The listing builds one solid part. Answer for the finished solid, in the listing's coordinates (mm). Coordinates: 2 decimals unless noted, no trailing zeros. Write each loop counter-clockwise with the first axis right and the second up, starting at its lowest first coordinate (ties: lowest second). Pieces come first, ordered by that corner, then holes.
(1) The part is cut by section A-A on z = 98. Give the number of separate pieces and of enclosed holes in the cut face, plus the area to 3 significant figures.
(2) The part is cut by section C-C on y = 48. Determine the outline of the cut face in (x, z).
(3) Straight lines are drawn through the part: line 1 (Y direction, x = 34.5, z = 41); line 2 (Z direction, x = 24, y = 36.5); line 3 (Y direction, x = -33, z = 49). For each, find the intervals that lie inside material, in ascending order.
(4) Given P1, Ø1.9, axis at x = 34, z = 52, coming from the -Y side; P2, Ø5, axis at x = 4, y = -36.5, coming from the -Z side; P3, Ø1.9, axis at x = 1, z = 97.5, coming from the +Y side, each flat-ended and moving along its own axis, determine where each tip first touches the part or whether it passes through.
(5) The part is cut by section B-B on x = 0. Determine the outline of the cut face in (y, z), plus the area to 3 significant figures.
Autodesk Fusion 360 part; units mm, degrees
sketch "Sketch1" plane through (0, 0, 0) normal (0, 0, 1) x (1, 0, 0)
  line L0 (63.5, 63.5) -> (-63.5, 63.5)
  line L1 (-63.5, 63.5) -> (-63.5, -63.5)
  line L2 (-63.5, -63.5) -> (63.5, -63.5)
  line L3 (63.5, -63.5) -> (63.5, 63.5)
  line L4 (63.5, 63.5) -> (-63.5, -63.5) construction
  line L5 (-63.5, 63.5) -> (63.5, -63.5) construction
extrude "Extrude1" add sketch "Sketch1" along normal blind 127
sketch "Sketch2" plane through (0, 0, 127) normal (0, 0, 1) x (-1, 0, 0)
  line L0 (-63.5, 63.5) -> (-63.5, -63.5)
  line L1 (-63.5, -63.5) -> (63.5, -63.5)
  line L2 (63.5, -63.5) -> (63.5, 63.5)
  line L3 (63.5, 63.5) -> (-63.5, 63.5)
  line L4 (31.75, 31.75) -> (-31.75, 31.75)
  line L5 (-31.75, 31.75) -> (-31.75, -31.75)
  line L6 (-31.75, -31.75) -> (31.75, -31.75)
  line L7 (31.75, -31.75) -> (31.75, 31.75)
  dimension "d3" = -31.75
sketch "Sketch3" plane through (0, -63.5, 0) normal (0, -1, 0) x (1, 0, 0)
  line L0 (-63.5, 0) -> (63.5, 0)
  line L1 (63.5, 0) -> (63.5, 127)
  line L2 (63.5, 127) -> (-63.5, 127)
  line L3 (-63.5, 127) -> (-63.5, 0)
  line L4 (-31.75, 31.75) -> (31.75, 31.75)
  line L5 (31.75, 31.75) -> (31.75, 95.25)
  line L6 (31.75, 95.25) -> (-31.75, 95.25)
  line L7 (-31.75, 95.25) -> (-31.75, 31.75)
  dimension "d4" = -31.75
sketch "Sketch4" plane through (0, 0, 0) normal (0, 0, -1) x (1, 0, 0)
  line L0 (63.5, -63.5) -> (63.5, 63.5)
  line L1 (63.5, 63.5) -> (-63.5, 63.5)
  line L2 (-63.5, 63.5) -> (-63.5, -63.5)
  line L3 (-63.5, -63.5) -> (63.5, -63.5)
sketch "Sketch5" plane through (-63.5, 0, 0) normal (-1, 0, 0) x (0, -1, 0)
  line L0 (-63.5, 0) -> (63.5, 0)
  line L1 (63.5, 0) -> (63.5, 127)
  line L2 (63.5, 127) -> (-63.5, 127)
  line L3 (-63.5, 127) -> (-63.5, 0)
  line L4 (-31.75, 31.75) -> (31.75, 31.75)
  line L5 (31.75, 31.75) -> (31.75, 95.25)
  line L6 (31.75, 95.25) -> (-31.75, 95.25)
  line L7 (-31.75, 95.25) -> (-31.75, 31.75)
  dimension "d5" = -31.75
extrude "Extrude2" cut sketch "Sketch2" against normal blind 127 contours L4 L5 L6 L7
extrude "Extrude3" cut sketch "Sketch5" against normal blind 127 contours L4 L5 L6 L7
extrude "Extrude4" cut sketch "Sketch3" against normal blind 127 contours L4 L5 L6 L7
chamfer "Chamfer1" distance 25.4 angle 45 4 edges at (0, -63.5, 95.25) (31.75, -63.5, 63.5) (0, -63.5, 31.75) (-31.75, -63.5, 63.5)
chamfer "Chamfer2" distance 25.4 angle 45 4 edges at (-63.5, 31.75, 63.5) (-63.5, 0, 95.25) (-63.5, -31.75, 63.5) (-63.5, 0, 31.75)
chamfer "Chamfer3" distance 25.4 angle 45 4 edges at (31.75, 63.5, 63.5) (0, 63.5, 95.25) (-31.75, 63.5, 63.5) (0, 63.5, 31.75)
chamfer "Chamfer4" distance 25.4 angle 45 4 edges at (63.5, 0, 95.25) (63.5, 31.75, 63.5) (63.5, 0, 31.75) (63.5, -31.75, 63.5)
chamfer "Chamfer5" distance 25.4 angle 45 4 edges at (-31.75, 0, 127) (0, 31.75, 127) (31.75, 0, 127) (0, -31.75, 127)
chamfer "Chamfer6" distance 25.4 angle 45 4 edges at (31.75, 0, 0) (0, 31.75, 0) (-31.75, 0, 0) (0, -31.75, 0)
extrude "Extrude5" cut 1 faces at (-55.0333, 10.5833, 112.1833) along direction (0.707107, 0, 0.707107) blind 12.7
extrude "Extrude6" cut 1 faces at (-55.0333, 10.5833, 14.8167) along direction (0.707107, 0, -0.707107) blind 12.7
extrude "Extrude7" cut 1 faces at (-10.5833, -55.0333, 14.8167) along direction (0, 0.707107, -0.707107) blind 12.7
extrude "Extrude8" cut 1 faces at (-10.5833, -55.0333, 112.1833) along direction (0, 0.707107, 0.707107) blind 12.7
extrude "Extrude9" cut 1 faces at (55.0333, 10.5833, 14.8167) along direction (-0.707107, 0, -0.707107) blind 12.7
extrude "Extrude10" cut 1 faces at (55.0333, -10.5833, 112.1833) along direction (-0.707107, 0, 0.707107) blind 12.7
extrude "Extrude11" cut 1 faces at (-10.5833, 55.0333, 14.8167) along direction (0, -0.707107, -0.707107) blind 12.7
extrude "Extrude12" cut 1 faces at (10.5833, 55.0333, 112.1833) along direction (0, -0.707107, 0.707107) blind 12.7
extrude "Extrude13" cut 1 faces at (48.6833, 55.0333, 74.0833) along direction (0.707107, -0.707107, 0) blind 12.7
extrude "Extrude14" cut 1 faces at (-48.6833, 55.0333, 74.0833) along direction (-0.707107, -0.707107, 0) blind 12.7
extrude "Extrude15" cut 1 faces at (-48.6833, -55.0333, 52.9167) along direction (-0.707107, 0.707107, 0) blind 12.7
extrude "Extrude16" cut 1 faces at (48.6833, -55.0333, 74.0833) along direction (0.707107, 0.707107, 0) blind 12.7
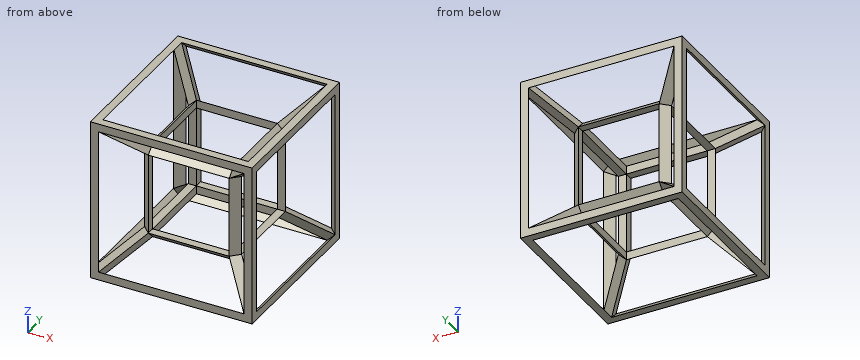
Model answer:
1. separate pieces: 5
1. enclosed holes: 1
1. area: 1,190 mm2
2. outline: (-63.5, 0) - (-57.15, 0) - (-63.5, 6.35) - close; (-63.5, 120.65) - (-57.15, 127) - (-63.5, 127) - close; (-54.35, 15.5) - (-48, 9.15) - (-41.65, 21.85) - close; (-54.35, 111.5) - (-41.65, 105.15) - (-48, 117.85) - close; (41.65, 21.85) - (48, 9.15) - (54.35, 15.5) - close; (41.65, 105.15) - (54.35, 111.5) - (48, 117.85) - close; (57.15, 0) - (63.5, 0) - (63.5, 6.35) - close; (57.15, 127) - (63.5, 120.65) - (63.5, 127) - close
3. line 1: y = -35.35 to -31.75, 31.75 to 35.35
3. line 2: z = 30.15 to 31.75, 95.25 to 96.85
3. line 3: y = -36.85 to -31.75, 31.75 to 36.85
4. P1: stops at y = -36.8
4. P2: stops at z = 27.65
4. P3: stops at y = 36.8
5. outline: (-63.5, 0) - (-57.15, 0) - (-63.5, 6.35) - close; (-63.5, 120.65) - (-57.15, 127) - (-63.5, 127) - close; (-38.1, 31.75) - (-31.75, 25.4) - (-31.75, 31.75) - close; (-38.1, 95.25) - (-31.75, 95.25) - (-31.75, 101.6) - close; (31.75, 25.4) - (38.1, 31.75) - (31.75, 31.75) - close; (31.75, 95.25) - (38.1, 95.25) - (31.75, 101.6) - close; (57.15, 0) - (63.5, 0) - (63.5, 6.35) - close; (57.15, 127) - (63.5, 120.65) - (63.5, 127) - close
5. area: 161 mm2
